```python
from build123d import *

# Parameters (mm, degrees)
SKETCH_1_W          = 30
SKETCH_1_H          = 180
EXTRUDE_1_DEPTH     = 12
SKETCH_2_R          = 5.5
CUT_EXTRUDE_1_DEPTH = 12
CHAMFER_1_SIZE      = 6


with BuildPart() as part:
    # 草图1 → 凸台-拉伸1 (new body)
    with BuildSketch(Plane.XY):
        Rectangle(SKETCH_1_W, SKETCH_1_H)
    extrude(amount=EXTRUDE_1_DEPTH)

    # 草图2 → 切除-拉伸1 (cut)
    with BuildSketch(Plane.XY.offset(12)):
        with Locations((0, -75)):
            Circle(SKETCH_2_R)
        with BuildLine():
            Line((4.5, 75), (4.5, -55))
            ThreePointArc((4.5, -55), (0, -59.5), (-4.5, -55))
            Line((-4.5, -55), (-4.5, 75))
            ThreePointArc((-4.5, 75), (0, 79.5), (4.5, 75))
        make_face()
    extrude(amount=-CUT_EXTRUDE_1_DEPTH, mode=Mode.SUBTRACT)

    # 倒角1
    chamfer_1_edges = [part.edges().sort_by_distance(p)[0] for p in [
        (-15, 90, 6),
    ]]
    chamfer(chamfer_1_edges, length=CHAMFER_1_SIZE)


solid = part.part
```
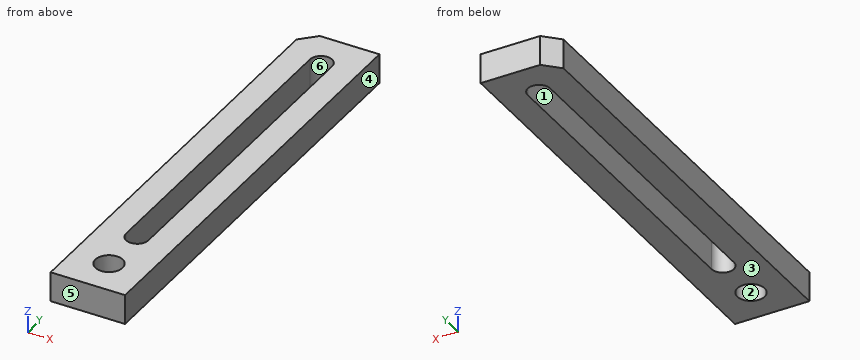
Model file for the job. Use its own axes, mm. Face numbers are marked on the shaded views. A direction names the side the tool comes from. Coordinates: 2 decimals unless noted, no trailing zeros. Write each loop counter-clockwise with the first axis right and the second up, starting at its lowest first coordinate (ties: lowest second). Pieces come first, ordered by that corner, then holes. Notation, with made-up numbers: (54.5, -20.5) - (63.5, -20.5) arc R18 cw to (63.5, 12.5) - close; hole circle Ø10 at (74.25, 73). An arc over 180 degrees is marked (long way). Use a Markdown table: item, result. Add a question column.
Item 1: Two-plate mould, pull along X, no slides. Class the marked faces 1, 2, 3 and 4: pulls with the +X half, pulls with the -X half, needs draft (parallel to the pull), parting line crosses it, or undercut.
Item 2: Band-saw the part on C-C, the plane z = 4.25. Write the cut outline in (x, y), and give its area (3 significant figures).
Item 3: Drill centre lines: line 1 along Y through (x, z) = (0, 8.25); line 2 along X through (y, z) = (52.5, 5); line 3 along Y through (x, z) = (3, 1). Where is each one in solid material? Low to high.
Item 4: Band-saw the part on A-A, the plane y = 63.5. Write the cut outline in (x, z), and give its area (3 significant figures).
Item 5: 3-axis set-ups, long thin cutter, end or side, ignore diameter. For the marked faces 5 and 6: which of +Z, -Z, +X, -X, +Y, -Y reach the whole face in a straight line?
Item 6: Band-saw the part on B-B, the plane x = 0. Write the cut outline in (y, z).
Item 7: Band-saw the part on D-D, the plane y = -75. Write the cut outline in (x, z), and give its area (3 significant figures).
A:
| question | item | result |
|---|---|---|
| 1 | face 1 | undercut |
| 1 | face 2 | undercut |
| 1 | face 3 | needs draft |
| 1 | face 4 | pulls with the +X half |
| 2 | outline | (-15, -90) - (15, -90) - (15, 90) - (-9, 90) - (-15, 84) - close; hole circle Ø11 at (0, -75); hole (-4.5, -55) arc R4.5 ccw to (4.5, -55) - (4.5, 75) arc R4.5 ccw to (-4.5, 75) - close |
| 2 | area | 4,050 mm² |
| 3 | line 1 | y = -90 to -80.5, -69.5 to -59.5, 79.5 to 90 |
| 3 | line 2 | x = -15 to -4.5, 4.5 to 15 |
| 3 | line 3 | y = -90 to -79.61, -70.39 to -58.35, 78.35 to 90 |
| 4 | outline | (-15, 0) - (-4.5, 0) - (-4.5, 12) - (-15, 12) - close; (4.5, 0) - (15, 0) - (15, 12) - (4.5, 12) - close |
| 4 | area | 252 mm² |
| 5 | face 5 | +Z, -Z, +X, -X, -Y |
| 5 | face 6 | +Z, -Z |
| 6 | outline | (-90, 0) - (-80.5, 0) - (-80.5, 12) - (-90, 12) - close; (-69.5, 0) - (-59.5, 0) - (-59.5, 12) - (-69.5, 12) - close; (79.5, 0) - (90, 0) - (90, 12) - (79.5, 12) - close |
| 7 | outline | (-15, 0) - (-5.5, 0) - (-5.5, 12) - (-15, 12) - close; (5.5, 0) - (15, 0) - (15, 12) - (5.5, 12) - close |
| 7 | area | 228 mm² |
